Can you work these out from the model? Positions are in its coordinate system, mm. A direction names the side the tool comes from. Round coordinates to 2 decimals unless told otherwise and drop trailing zeros. Loops run counter-clockwise (first coordinate to the right, second up) from the corner with the lowest first, then second, coordinate; pieces in that order, holes last. Notation, with made-up numbers: M 58.5,-31 L 88.5,-31 A19 ccw 88.5,1 Z; hole C 53.25,6 d9. An arc over 180 degrees is marked long. Answer as CSV lines item,"result".
from build123d import *

# Parameters (mm, degrees)
CROQUIS1_R              = 7.5
SALIENTE_EXTRUIR1_DEPTH = 20
SALIENTE_EXTRUIR2_DEPTH = 45
SALIENTE_EXTRUIR3_DEPTH = 75
CROQUIS2_R              = 6
CORTAR_EXTRUIR1_DEPTH   = 75


with BuildPart() as part:
    # Croquis1 → Saliente-Extruir1 (new body)
    with BuildSketch(Plane.XY):
        with BuildLine():
            Line((29.047375097, 7.5), (-29.047375097, 7.5))
            ThreePointArc((-29.047375097, 7.5), (-27.171188586, 12.717173855), (-24.366985862, 17.5))
            ThreePointArc((-24.366985862, 17.5), (-16.360726635, 25.146105543), (-6.126443354, 29.36778323))
            Line((-6.126443354, 29.36778323), (-75, 15))
            ThreePointArc((-75, 15), (-90, 0), (-75, -15))
            Line((-75, -15), (-6.126443354, -29.36778323))
            ThreePointArc((-6.126443354, -29.36778323), (-16.360726635, -25.146105543), (-24.366985862, -17.5))
            ThreePointArc((-24.366985862, -17.5), (-27.171188586, -12.717173855), (-29.047375097, -7.5))
            Line((-29.047375097, -7.5), (29.047375097, -7.5))
            ThreePointArc((29.047375097, -7.5), (27.171188586, -12.717173855), (24.366985862, -17.5))
            ThreePointArc((24.366985862, -17.5), (16.360726635, -25.146105543), (6.126443354, -29.36778323))
            Line((6.126443354, -29.36778323), (75, -15))
            ThreePointArc((75, -15), (90, 0), (75, 15))
            Line((75, 15), (6.126443354, 29.36778323))
            ThreePointArc((6.126443354, 29.36778323), (16.360726635, 25.146105543), (24.366985862, 17.5))
            ThreePointArc((24.366985862, 17.5), (27.171188586, 12.717173855), (29.047375097, 7.5))
        make_face()
        with Locations((-75, 0)):
            Circle(CROQUIS1_R, mode=Mode.SUBTRACT)
        with Locations((75, 0)):
            Circle(CROQUIS1_R, mode=Mode.SUBTRACT)
    extrude(amount=SALIENTE_EXTRUIR1_DEPTH)

    # Croquis1<3> → Saliente-Extruir2 (add)
    with BuildSketch(Plane.XY):
        with BuildLine():
            ThreePointArc((24.366985862, 17.5), (0, 30), (-24.366985862, 17.5))
            Line((-24.366985862, 17.5), (24.366985862, 17.5))
        make_face()
        with BuildLine():
            ThreePointArc((-24.366985862, -17.5), (0, -30), (24.366985862, -17.5))
            Line((24.366985862, -17.5), (-24.366985862, -17.5))
        make_face()
    extrude(amount=SALIENTE_EXTRUIR2_DEPTH)

    # Croquis1<4> → Saliente-Extruir3 (add)
    with BuildSketch(Plane.XY):
        with BuildLine():
            ThreePointArc((-24.366985862, 17.5), (-27.171188586, 12.717173855), (-29.047375097, 7.5))
            Line((-29.047375097, 7.5), (29.047375097, 7.5))
            ThreePointArc((29.047375097, 7.5), (27.171188586, 12.717173855), (24.366985862, 17.5))
            Line((24.366985862, 17.5), (-24.366985862, 17.5))
        make_face()
        with BuildLine():
            ThreePointArc((-29.047375097, -7.5), (-27.171188586, -12.717173855), (-24.366985862, -17.5))
            Line((-24.366985862, -17.5), (24.366985862, -17.5))
            ThreePointArc((24.366985862, -17.5), (27.171188586, -12.717173855), (29.047375097, -7.5))
            Line((29.047375097, -7.5), (-29.047375097, -7.5))
        make_face()
    extrude(amount=SALIENTE_EXTRUIR3_DEPTH)

    # Croquis2 → Cortar-Extruir1 (cut)
    with BuildSketch(Plane.XZ.offset(17.5)):
        with Locations((0, 60)):
            Circle(CROQUIS2_R)
    extrude(amount=-CORTAR_EXTRUIR1_DEPTH, mode=Mode.SUBTRACT)


solid = part.part
Item 1: Will these pins go through, and if not, where does the flat tip stop? pin 1 (1 mm diameter, centred on y = 11.5, z = 49.5, fed in from -X); pin 2 (11 mm diameter, centred on x = 0, z = 60, fed in from -Y); pin 3 (15 mm diameter, centred on x = -12, z = 53, fed in from -Y); pin 4 (2 mm diameter, centred on y = -1.5, z = 10, fed in from -X).
Output:
pin 1,"stops at x = -27.91"
pin 2,"passes through"
pin 3,"stops at y = -17.5"
pin 4,"stops at x = -89.99"
Item 2: We'd pull the mould along Y, two halves only. Please class faces 1 (the face through (-41.045, -22.083, 9.86)), 2 (the face through (0, -7.5, 47)), 3 (the face through (-4.42, -12.57, 64.06)): released by +Y, released by -Y, zero draft, split by the parting line, or undercut.
Output:
face 1,"released by -Y"
face 2,"undercut"
face 3,"zero draft"
Item 3: If we section it at C-C on z = 60: Write out the boundary of the cut face in (x, y), then the cut area to 3 significant figures.
Output:
outline,"M -29.05,-7.5 A30 ccw -24.37,-17.5 L -6,-17.5 L -6,-7.5 Z; M -29.05,7.5 L -6,7.5 L -6,17.5 L -24.37,17.5 A30 ccw Z; M 6,-17.5 L 24.37,-17.5 A30 ccw 29.05,-7.5 L 6,-7.5 Z; M 6,7.5 L 29.05,7.5 A30 ccw 24.37,17.5 L 6,17.5 Z"
area,"843 mm2"
Item 4: If we section it at B-B on z = 23.5: Write out the boundary of the cut face in (x, y).
Output:
outline,"M -29.05,-7.5 A30 ccw 29.05,-7.5 Z; M -29.05,7.5 L 29.05,7.5 A30 ccw Z"
Item 5: If we section it at A-A on x = 0: Write out the boundary of the cut face in (y, z).
Output:
outline,"M -30,0 L 30,0 L 30,45 L 17.5,45 L 17.5,54 L 7.5,54 L 7.5,20 L -7.5,20 L -7.5,54 L -17.5,54 L -17.5,45 L -30,45 Z; M -17.5,66 L -7.5,66 L -7.5,75 L -17.5,75 Z; M 7.5,66 L 17.5,66 L 17.5,75 L 7.5,75 Z"
Item 6: If we section it at D-D on y = 0: Write out the boundary of the cut face in (x, z).
Output:
outline,"M -90,0 L -82.5,0 L -82.5,20 L -90,20 Z; M -67.5,0 L 67.5,0 L 67.5,20 L -67.5,20 Z; M 82.5,0 L 90,0 L 90,20 L 82.5,20 Z"
Item 7: If I drill on line 1 along X through (y, z) = (-0.5, 10); line 2 along Y through (x, z) = (7.5, 64); line 3 along Z through (x, y) = (0, 12.5), over which ranges is the centre line in solid material (lowest first)? Write a range as from..to.
Output:
line 1,"x = -89.99..-82.48, -67.52..67.52, 82.48..89.99"
line 2,"y = -17.5..-7.5, 7.5..17.5"
line 3,"z = 0..54, 66..75"
Item 8: On a 3-axis mill with a long thin cutter (end or side, diameter ignored), from which of +Z, -Z, +X, -X, +Y, -Y can I reach the whole of each face in a straight line? I mean faces 4 (the face through (0, 7.5, 47)), 5 (the face through (0, -22, 45)), 6 (the face through (6, 17.5, 56)), 7 (the face through (-1, 0, 20)), 8 (the face through (90, 0, 10)). Say none if no direction works.
Output:
face 4,"+Z, +X, -X"
face 5,"+Z, +X, -X, -Y"
face 6,"+Z, +X, -X, +Y"
face 7,"+Z"
face 8,"+Z, -Z, +X"
